from build123d import *

# Parameters (mm, degrees)
SKETCH1_W           = 52
SKETCH1_H           = 33.3
COVER_PLATE_DEPTH   = 3
SKETCH2_W           = 5
SKETCH2_H           = 14.8
SKETCH2_W_2         = 7
SKETCH2_H_2         = 16.8
CABLE_NOTCHES_DEPTH = 5
SKETCH3_R           = 1.7
SCREW_HOLES_DEPTH   = 5


with BuildPart() as part:
    # Sketch1 → Cover Plate (new body)
    with BuildSketch(Plane.XY.offset(124.4)):
        with Locations((-36.5, -10.15)):
            Rectangle(SKETCH1_W, SKETCH1_H)
    extrude(amount=COVER_PLATE_DEPTH)

    # Sketch2 → Cable Notches (cut)
    with BuildSketch(Plane.XY.offset(123.4)):
        with Locations((-43.8, -20.4)):
            Rectangle(SKETCH2_W, SKETCH2_H)
        with Locations((-29.2, -19.4)):
            Rectangle(SKETCH2_W_2, SKETCH2_H_2)
    extrude(amount=CABLE_NOTCHES_DEPTH, mode=Mode.SUBTRACT)

    # Sketch3 → Screw Holes (cut)
    with BuildSketch(Plane.XY.offset(123.4)):
        with Locations((-57, -22.3)):
            Circle(SKETCH3_R)
        with Locations((-57, 2.5)):
            Circle(SKETCH3_R)
        with Locations((-16, -22.3)):
            Circle(SKETCH3_R)
        with Locations((-16, 2.5)):
            Circle(SKETCH3_R)
    extrude(amount=SCREW_HOLES_DEPTH, mode=Mode.SUBTRACT)


solid = part.part
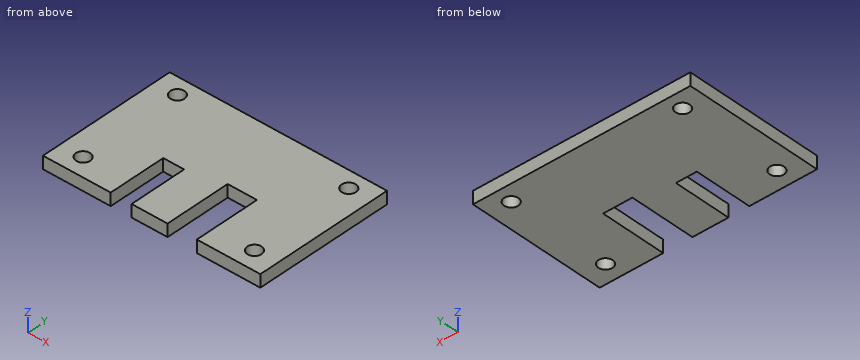
Geometry check sheet. Reference: the model listing, model coordinates, mm. Round coordinates to 2 decimals unless told otherwise and drop trailing zeros. Order: outer loops, then holes, each group sorted by start corner. A loop starts at its lowest first (then second) coordinate and runs counter-clockwise, first axis right, second up. Notation, with made-up numbers: (-23, -28.75) -> (-12, -28.75) arc R15 cw to (-12, -0.75) -> close; hole circle Ø10 at (9.5, 11.5). An arc over 180 degrees is marked (long way). Use one line per item in the form item = value.
1. Cross-section at A-A, the plane z = 125.05. Enter the section's corners in (x, y).
Working result:
outline = (-62.5, -26.8) -> (-46.3, -26.8) -> (-46.3, -13) -> (-41.3, -13) -> (-41.3, -26.8) -> (-32.7, -26.8) -> (-32.7, -11) -> (-25.7, -11) -> (-25.7, -26.8) -> (-10.5, -26.8) -> (-10.5, 6.5) -> (-62.5, 6.5) -> close; hole circle Ø3.4 at (-57, -22.3); hole circle Ø3.4 at (-57, 2.5); hole circle Ø3.4 at (-16, -22.3); hole circle Ø3.4 at (-16, 2.5)
2. Cross-section at D-D, the plane y = -22.3. Enter the section's corners in (x, z).
Working result:
outline = (-62.5, 124.4) -> (-58.7, 124.4) -> (-58.7, 127.4) -> (-62.5, 127.4) -> close; (-55.3, 124.4) -> (-46.3, 124.4) -> (-46.3, 127.4) -> (-55.3, 127.4) -> close; (-41.3, 124.4) -> (-32.7, 124.4) -> (-32.7, 127.4) -> (-41.3, 127.4) -> close; (-25.7, 124.4) -> (-17.7, 124.4) -> (-17.7, 127.4) -> (-25.7, 127.4) -> close; (-14.3, 124.4) -> (-10.5, 124.4) -> (-10.5, 127.4) -> (-14.3, 127.4) -> close
3. Scan lines: line 1 along X through (y, z) = (2.5, 125.1); line 2 along X through (y, z) = (-20, 125); line 3 along X through (y, z) = (-22.3, 125.75). Record each from-to range of solid material in increasing order. Write a range as from..to.
Working result:
line_1 = -62.5..-58.7, -55.3..-17.7, -14.3..-10.5
line_2 = -62.5..-46.3, -41.3..-32.7, -25.7..-10.5
line_3 = -62.5..-58.7, -55.3..-46.3, -41.3..-32.7, -25.7..-17.7, -14.3..-10.5
4. Go/stop test with flat-tipped pins: pin 1 (0.9 mm diameter, centred on x = -31, z = 126.5, fed in from -Y); pin 2 (1.5 mm diameter, centred on x = -43.5, z = 126, fed in from -Y). Record where each tip stops, or that it passes through.
Working result:
pin_1 = -11
pin_2 = -13
5. Cross-section at B-B, the plane y = -15.5. Enter the section's corners in (x, z), plus the area to 3 significant figures.
Working result:
outline = (-62.5, 124.4) -> (-46.3, 124.4) -> (-46.3, 127.4) -> (-62.5, 127.4) -> close; (-41.3, 124.4) -> (-32.7, 124.4) -> (-32.7, 127.4) -> (-41.3, 127.4) -> close; (-25.7, 124.4) -> (-10.5, 124.4) -> (-10.5, 127.4) -> (-25.7, 127.4) -> close
area = 120 mm^2
6. Cross-section at C-C, the plane x = -16. Enter the section's corners in (y, z), plus the area to 3 significant figures.
Working result:
outline = (-26.8, 124.4) -> (-24, 124.4) -> (-24, 127.4) -> (-26.8, 127.4) -> close; (-20.6, 124.4) -> (0.8, 124.4) -> (0.8, 127.4) -> (-20.6, 127.4) -> close; (4.2, 124.4) -> (6.5, 124.4) -> (6.5, 127.4) -> (4.2, 127.4) -> close
area = 79.5 mm^2
